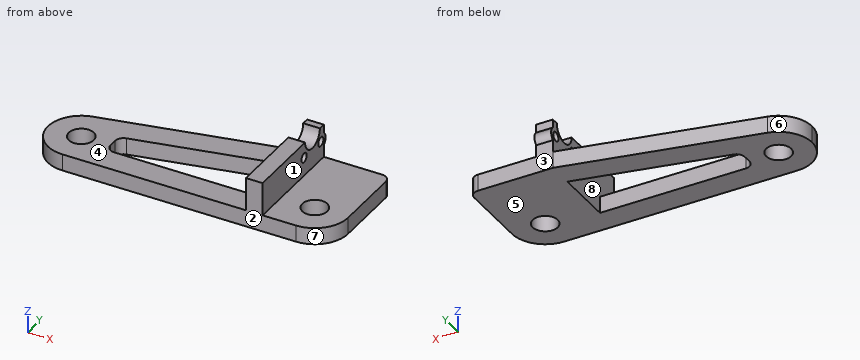
```python
from build123d import *

# Parameters (mm, degrees)
F0_R      = 4.7625
F1_DEPTH  = 6.35
F2_R      = 12.69999
F3_W      = 6.35
F3_H      = 41.275
F4_DEPTH  = 12.7
F6_DEPTH  = 25.4
F7_R      = 3.175
F8_R      = 5.0038
F8_R_2    = 1.7526
F9_DEPTH  = 25.4
F11_DEPTH = 6.35


# Not quite as in the source:
# - a fillet or chamfer is up to 0.001 mm smaller than in the source, because OpenCascade refuses the exact size


with BuildPart() as f1:
    # F0 (on Top) → F1 (new body)
    with BuildSketch(Plane.XY):
        Polygon((-101.6, -12.7), (12.7, -12.7), (12.7, 28.575), (-19.05, 28.575), (-101.6, 10.1816951473), align=None)
        with Locations((-88.9, 0)):
            Circle(F0_R, mode=Mode.SUBTRACT)
        Circle(F0_R, mode=Mode.SUBTRACT)
    extrude(amount=F1_DEPTH)

    # F2 (radius 12.7 in the source; OpenCascade refuses exactly that, so slightly less here)
    f2_edges = [f1.edges().sort_by_distance(p)[0] for p in [
        (12.7, -12.7, 3.175),
        (-101.6, -12.7, 3.175),
        (-101.6, 10.181695, 3.175),
    ]]
    fillet(f2_edges, radius=F2_R)

    # F3 (on face) → F4 (join)
    with BuildSketch(Plane.XY.offset(6.35)):
        with Locations((-15.875, 7.9375)):
            Rectangle(F3_W, F3_H)
    extrude(amount=F4_DEPTH)

    # F5 (on face) → F6 (cut)
    with BuildSketch(Plane.XY.offset(6.35)):
        with BuildLine():
            Line((-19.05, 18.8164242334), (-75.3030020415, 6.2824615995))
            ThreePointArc((-75.3030020415, 6.2824615995), (-77.0896928651, 5.1694426385), (-77.7875, 3.1834566091))
            Line((-77.7875, 3.1834566091), (-77.7875, 0))
            ThreePointArc((-77.7875, 0), (-76.8575640303, -2.2450640303), (-74.6125, -3.175))
            Line((-74.6125, -3.175), (-19.05, -3.175))
            Line((-19.05, -3.175), (-19.05, 18.8164242334))
        make_face()
    extrude(amount=-F6_DEPTH, mode=Mode.SUBTRACT)

    # F7
    f7_edges = [f1.edges().sort_by_distance(p)[0] for p in [
        (12.7, 28.575, 3.175),
    ]]
    fillet(f7_edges, radius=F7_R)

    # F8 (on face) → F9 (cut)
    with BuildSketch(Plane.YZ.offset(-12.7)):
        with Locations((20.955, 19.05)):
            Circle(F8_R)
        with Locations((26.6065, 13.3985)):
            Circle(F8_R_2)
        with Locations((15.3035, 13.3985)):
            Circle(F8_R_2)
    extrude(amount=-F9_DEPTH, mode=Mode.SUBTRACT)

    # F10 (on face) → F11 (join)
    with BuildSketch(Plane.YZ.offset(-12.7)):
        with BuildLine():
            Line((28.575, 15.8896107462), (28.575, 10.9073892538))
            ThreePointArc((28.575, 10.9073892538), (29.7815, 13.3985), (28.575, 15.8896107462))
        make_face()
    extrude(amount=-F11_DEPTH)


solid = f1.part
```
Can you work these out from the model? Positions are in its coordinate system, mm. Face numbers are marked on the shaded views. A direction names the side the tool comes from. Coordinates: 2 decimals unless noted, no trailing zeros. Write each loop counter-clockwise with the first axis right and the second up, starting at its lowest first coordinate (ties: lowest second). Pieces come first, ordered by that corner, then holes. Notation, with made-up numbers: (31.5, 24) - (50.5, 24) arc R20 ccw to (50.5, 33) - close; hole circle Ø2 at (28.5, 65.5). An arc over 180 degrees is marked (long way). Return JSON: item names as keys, results as strings.
Q1. If we section it at D-D (y = 21): Please give me the cut outline in (x, z), then the cut area to 3 significant figures.
Computed values:
{"outline": "(-53.05, 0) - (12.7, 0) - (12.7, 6.35) - (-12.7, 6.35) - (-12.7, 14.05) - (-19.05, 14.05) - (-19.05, 6.35) - (-53.05, 6.35) - close", "area": "466 mm2"}
Q2. Thinking about a two-plate mould opening in X: for the marked faces 6, 7 and 8, which applies, +X half, -X half, draft (parallel to the pull), parting line (faces both ways), or undercut?
Computed values:
{"face 6": "-X half", "face 7": "+X half", "face 8": "undercut"}
Q3. On a 3-axis mill with a long thin cutter (end or side, diameter ignored), from which of +Z, -Z, +X, -X, +Y, -Y can I reach the whole of each face in a straight line? I mean the marked faces 1, 2, 3, 4 and 5. Say none if no direction works.
Computed values:
{"face 1": "+Z, +X, +Y, -Y", "face 2": "+Z, -Z, +X, -X, -Y", "face 3": "-Z, +X, -X, +Y", "face 4": "+Z, -X, +Y, -Y", "face 5": "-Z, +X, -X, +Y, -Y"}
Q4. If we section it at B-B (x = -61): Please give me the cut outline in (y, z) (3 decimals).
Computed values:
{"outline": "(-12.7, 0) - (-3.175, 0) - (-3.175, 6.35) - (-12.7, 6.35) - close; (9.469, 0) - (19.228, 0) - (19.228, 6.35) - (9.469, 6.35) - close"}
Q5. I'm going to push flat-ended pins straight in: pin 1 Ø0.9 at (x, z) = (-16, 16.5) entering from +Y (3 decimals); pin 2 Ø1.5 at (x, y) = (-38, 21) entering from +Z; pin 3 Ø4 at (y, z) = (15.3, 13.4) entering from +X; pin 4 Ø8.5 at (x, y) = (-88.9, 0) entering from +Z. Where does each tip first touch, or does it pass through?
Computed values:
{"pin 1": "stops at y = 28.575", "pin 2": "stops at z = 6.35", "pin 3": "stops at x = -12.7", "pin 4": "passes through"}
Q6. Please list where these lines run through material, in increasing order: L1, parallel to Y at x = -6, z = 2.5 (3 decimals); L2, parallel to Z at x = 3.5, y = 28.5; L3, parallel to X at y = 10.5, z = 11.5. Write a range as from..to.
Computed values:
{"L1": "y = -12.7..28.575", "L2": "z = 0..6.35", "L3": "x = -19.05..-12.7"}
Q7. If we section it at A-A (z = 4): Count the separate pieces of the cut face and the enclosed holes in it, then the cut area to 3 significant figures.
Computed values:
{"separate pieces": "1", "enclosed holes": "3", "area": "2,820 mm2"}
